Can you work these out from the model? Positions are in its coordinate system, mm. Round coordinates to 2 decimals unless told otherwise and drop trailing zeros. Write each loop counter-clockwise with the first axis right and the second up, starting at its lowest first coordinate (ties: lowest second). Pieces come first, ordered by that corner, then holes. Notation, with made-up numbers: M 48.25,50 L 58.25,50 A24 cw 58.25,75 Z; hole C 66,37.5 d10. An arc over 180 degrees is marked long. Answer as a JSON object with one key per item and string values. Group by question number.
1) I'm going to push a flat-ended pin straight in: pin 1 Ø6 at (x, y) = (29.1, 36.525) entering from +Z. Where does the tip first touch, or does it pass through?
2) Suppose I cut it at C-C, the plane x = 50.1. Write out the boundary of the cut face in (y, z) (3 decimals), and give its area (3 significant figures).
3) Suppose I cut it at D-D, the plane z = 1.8. State how many separate pieces and enclosed holes the cut face has, and give its area (3 significant figures).
4) Suppose I cut it at B-B, the plane x = 29.1. Write out the boundary of the cut face in (y, z) (3 decimals).
5) Suppose I cut it at A-A, the plane x = 41.1. Write out the boundary of the cut face in (y, z) (1 decimal).
6) Please list where these lines run through material, in increasing order: L1, parallel to Y at x = 29.1, z = 1.5 (3 decimals); L2, parallel to Y at x = 41.1, z = 1.7 (1 decimal); L3, parallel to Y at x = 50.8, z = 0.75 (3 decimals). Write a range as [from, to].
from build123d import *

# Parameters (mm, degrees)
SKETCH1_R                  = 2.38125
BOSS_EXTRUDE1_DEPTH        = 2.54
M3_5_CLEARANCE_HOLE1_D     = 3.9
M3_5_CLEARANCE_HOLE1_DEPTH = 12.7
M3_5_CLEARANCE_HOLE1_TIP   = 1.171678207
SKETCH5_R                  = 4.7625
CUT_EXTRUDE1_DEPTH         = 71.688752465


with BuildPart() as part:
    # Sketch1 → Boss-Extrude1 (new body)
    with BuildSketch(Plane.XY):
        Polygon((-6.35, 9.525), (23.496082005, 41.525), (57.15, 41.525), (57.15, 0), (44.45, 0), (6.35, 0), (-6.35, 0), align=None)
        with Locations((0, 4.7625)):
            Circle(SKETCH1_R, mode=Mode.SUBTRACT)
        with Locations((50.8, 4.7625)):
            Circle(SKETCH1_R, mode=Mode.SUBTRACT)
    extrude(amount=BOSS_EXTRUDE1_DEPTH)

    # M3.5 Clearance Hole1
    with Locations(Plane.XY.offset(2.54)):
        with Locations((29.1, 36.525), (50.1, 36.525), (50.1, 14.525), (29.1, 14.525)):
            Hole(M3_5_CLEARANCE_HOLE1_D / 2, depth=M3_5_CLEARANCE_HOLE1_DEPTH)
            with Locations((0, 0, -(M3_5_CLEARANCE_HOLE1_DEPTH + M3_5_CLEARANCE_HOLE1_TIP / 2))):  # 118° drill point
                Cone(0, M3_5_CLEARANCE_HOLE1_D / 2, M3_5_CLEARANCE_HOLE1_TIP, mode=Mode.SUBTRACT)

    # Sketch5 → Cut-Extrude1 (cut, through all)
    with BuildSketch(Plane.XY.offset(2.54)):
        with Locations((41.1, 25.525)):
            Circle(SKETCH5_R)
    extrude(amount=-CUT_EXTRUDE1_DEPTH, mode=Mode.SUBTRACT)


solid = part.part
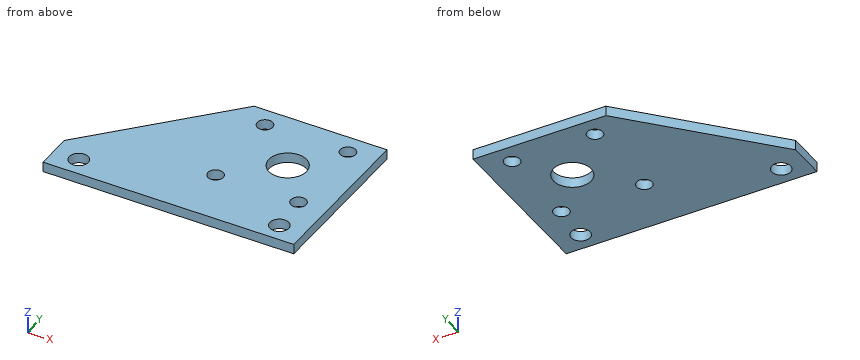
Results:
{
 "1": {"pin 1": "z = 2.54"},
 "2": {"outline": "M 0,0 L 2.486,0 L 2.486,2.54 L 0,2.54 Z; M 7.039,0 L 12.575,0 L 12.575,2.54 L 7.039,2.54 Z; M 16.475,0 L 34.575,0 L 34.575,2.54 L 16.475,2.54 Z; M 38.475,0 L 41.525,0 L 41.525,2.54 L 38.475,2.54 Z", "area": "74.1 mm^2"},
 "3": {"separate pieces": "1", "enclosed holes": "7", "area": "2,000 mm^2"},
 "4": {"outline": "M 0,0 L 12.575,0 L 12.575,2.54 L 0,2.54 Z; M 16.475,0 L 34.575,0 L 34.575,2.54 L 16.475,2.54 Z; M 38.475,0 L 41.525,0 L 41.525,2.54 L 38.475,2.54 Z"},
 "5": {"outline": "M 0,0 L 20.8,0 L 20.8,2.5 L 0,2.5 Z; M 30.3,0 L 41.5,0 L 41.5,2.5 L 30.3,2.5 Z"},
 "6": {"L1": "[0, 12.575], [16.475, 34.575], [38.475, 41.525]", "L2": "[0, 20.8], [30.3, 41.5]", "L3": "[0, 2.381], [7.144, 12.705], [16.345, 34.705], [38.345, 41.525]"}
}
